```python
from build123d import *

# Parameters (mm, degrees)
SKETCH1_R           = 1
BOSS_EXTRUDE1_DEPTH = 2
SKETCH2_R           = 4
SKETCH2_R_2         = 2.95
BOSS_EXTRUDE2_DEPTH = 5


with BuildPart() as part:
    # Sketch1 → Boss-Extrude1 (new body)
    with BuildSketch(Plane(origin=(0, 0, 0), x_dir=(1, 0, 0), z_dir=(0, 1, 0))):
        with BuildLine():
            Line((2.5, 20), (2.5, 7.5))
            ThreePointArc((2.5, 7.5), (3.964466094, 3.964466094), (7.5, 2.5))
            Line((7.5, 2.5), (20, 2.5))
            ThreePointArc((20, 2.5), (22.5, 0), (20, -2.5))
            Line((20, -2.5), (7.5, -2.5))
            ThreePointArc((7.5, -2.5), (3.964466094, -3.964466094), (2.5, -7.5))
            Line((2.5, -7.5), (2.5, -20))
            ThreePointArc((2.5, -20), (0, -22.5), (-2.5, -20))
            Line((-2.5, -20), (-2.5, -7.5))
            ThreePointArc((-2.5, -7.5), (-3.964466094, -3.964466094), (-7.5, -2.5))
            Line((-7.5, -2.5), (-20, -2.5))
            ThreePointArc((-20, -2.5), (-22.5, 0), (-20, 2.5))
            Line((-20, 2.5), (-7.5, 2.5))
            ThreePointArc((-7.5, 2.5), (-3.964466094, 3.964466094), (-2.5, 7.5))
            Line((-2.5, 7.5), (-2.5, 20))
            ThreePointArc((-2.5, 20), (0, 22.5), (2.5, 20))
        make_face()
        with Locations(Location((8.5, 0, 0), (0, 0, 270))):
            Circle(SKETCH1_R, mode=Mode.SUBTRACT)
    extrude(amount=BOSS_EXTRUDE1_DEPTH)

    # Sketch2 → Boss-Extrude2 (add)
    with BuildSketch(Plane.XZ):
        with Locations(Location((0, 0, 0), (0, 0, 90))):
            Circle(SKETCH2_R)
        with Locations(Location((0, 0, 0), (0, 0, 270))):
            Circle(SKETCH2_R_2, mode=Mode.SUBTRACT)
    extrude(amount=BOSS_EXTRUDE2_DEPTH)


solid = part.part
```
CAD build for the part. Positions are in the model's coordinates, mm. A direction names the side the tool comes from. Round coordinates to 2 decimals unless told otherwise and drop trailing zeros. Loops run counter-clockwise (first coordinate to the right, second up) from the corner with the lowest first, then second, coordinate; pieces in that order, holes last. Notation, with made-up numbers: (-17.5, 58) - (34.5, 58) arc R15 cw to (34.5, 65) - close; hole circle Ø10 at (86, 76.5). An arc over 180 degrees is marked (long way). Return JSON: item names as keys, results as strings. Group by question number.
Q1. Tool access for faces 1 (the face through (-2.88, -2.46, 0.64)), 2 (the face through (-2.5, 1, 14)), 3 (the face through (-2.5, 1, -14)), 4 (the face through (2.5, 1, 14)): list every direction of +Z, -Z, +X, -X, +Y, -Y with a clear straight run to the whole face (end or side of a thin tool).
Q2. Drill centre lines: line 1 along X through (y, z) = (-1.8, 0); line 2 along X through (y, z) = (0.6, 0); line 3 along Z through (x, y) = (-9, 1.25). Where is each one in solid material? Low to high. Write a range as [from, to].
Q3. Two-plate mould, pull along Z, no slides. Class faces 5 (the face through (14, 1, 2.5)), 6 (the face through (3.93, 0.99, -4)), 7 (the face through (-3, 0, 3)), 8 (the face through (0, 0, 0)): +Z half, -Z half, draft (parallel to the pull), parting line (faces both ways), or undercut.
Q4. Flat gauge pins, fed straight in: pin 1 Ø0.6 at (x, y) = (15, 1) entering from -Z; pin 2 Ø1.5 at (x, z) = (-2.5, 0) entering from -Y; pin 3 Ø2 at (x, y) = (16, 1) entering from +Z; pin 4 Ø1.6 at (y, z) = (0.5, -11.5) entering from -X. Where does each tip first touch, or does it go through?
Q5. Band-saw the part on D-D on z = -5.5. Give the cut face in (x, y), plus the area to 3 significant figures.
Q6. Band-saw the part on C-C on x = 0. Give the cut face in (y, z), plus the area to 4 significant figures.
Q7. Band-saw the part on A-A on y = 1. Give the cut face in (x, z).
Q8. Band-saw the part on B-B on x = 8.5. Give the cut face in (y, z), plus the area to 3 significant figures.
Solutions:
{
 "1": {"face 1": "-Y", "face 2": "+Z, -X, +Y, -Y", "face 3": "-Z, -X, +Y, -Y", "face 4": "+Z, +X, +Y, -Y"},
 "2": {"line 1": "x = [-4, -2.95], [2.95, 4]", "line 2": "x = [-22.5, 7.5], [9.5, 22.5]", "line 3": "z = [-2.5, 2.5]"},
 "3": {"face 5": "+Z half", "face 6": "-Z half", "face 7": "draft", "face 8": "undercut"},
 "4": {"pin 1": "stops at z = -2.5", "pin 2": "stops at y = -5", "pin 3": "stops at z = 2.5", "pin 4": "stops at x = -2.5"},
 "5": {"outline": "(-2.92, 0) - (2.92, 0) - (2.92, 2) - (-2.92, 2) - close", "area": "11.7 mm^2"},
 "6": {"outline": "(-5, -4) - (0, -4) - (0, -22.5) - (2, -22.5) - (2, 22.5) - (0, 22.5) - (0, 4) - (-5, 4) - (-5, 2.95) - (0, 2.95) - (0, -2.95) - (-5, -2.95) - close", "area": "100.5 mm^2"},
 "7": {"outline": "(-20, -2.5) - (-7.5, -2.5) arc R5 cw to (-2.5, -7.5) - (-2.5, -20) arc R2.5 ccw to (2.5, -20) - (2.5, -7.5) arc R5 cw to (7.5, -2.5) - (20, -2.5) arc R2.5 ccw to (20, 2.5) - (7.5, 2.5) arc R5 cw to (2.5, 7.5) - (2.5, 20) arc R2.5 ccw to (-2.5, 20) - (-2.5, 7.5) arc R5 cw to (-7.5, 2.5) - (-20, 2.5) arc R2.5 ccw to start; hole circle Ø2 at (8.5, 0)"},
 "8": {"outline": "(0, -2.5) - (2, -2.5) - (2, -1) - (0, -1) - close; (0, 1) - (2, 1) - (2, 2.5) - (0, 2.5) - close", "area": "6.00 mm^2"}
}
